Build history of the part. All positions in model axes, mm. Round coordinates to 2 decimals unless told otherwise and drop trailing zeros. Write each loop counter-clockwise with the first axis right and the second up, starting at its lowest first coordinate (ties: lowest second). Pieces come first, ordered by that corner, then holes.
from build123d import *

# Parameters (mm, degrees)
F0_W     = 25.4
F0_H     = 25.4
F0_W_2   = 22.098
F0_H_2   = 22.098
F1_DEPTH = 2133.6
F3_DEPTH = 25.401
F5_DEPTH = 25.401


with BuildPart() as f1:
    # F0 (on Right) → F1 (new body)
    with BuildSketch(Plane.YZ):
        with Locations((12.7, 12.7)):
            Rectangle(F0_W, F0_H)
        with Locations((12.7, 12.7)):
            Rectangle(F0_W_2, F0_H_2, mode=Mode.SUBTRACT)
    extrude(amount=F1_DEPTH)

    # F2 (on face) → F3 (cut, through all)
    with BuildSketch(Plane.XY.offset(25.4)):
        Polygon((2108.2, 25.4), (2133.6, 0), (2133.6, 25.4), align=None)
    extrude(amount=-F3_DEPTH, mode=Mode.SUBTRACT)

    # F4 (on face) → F5 (cut, through all)
    with BuildSketch(Plane.XY.offset(25.4)):
        Polygon((0, 25.4), (0, 0), (25.4, 25.4), align=None)
    extrude(amount=-F5_DEPTH, mode=Mode.SUBTRACT)


solid = f1.part
1) Slice it at A-A (y = 14). Write the cut outline in (x, z).
Results:
outline: (14, 0) - (2119.6, 0) - (2119.6, 1.65) - (14, 1.65) - close; (14, 23.75) - (2119.6, 23.75) - (2119.6, 25.4) - (14, 25.4) - close
2) Slice it at B-B (x = 1838.5). Write the cut outline in (y, z).
Results:
outline: (0, 0) - (25.4, 0) - (25.4, 25.4) - (0, 25.4) - close; hole (1.65, 1.65) - (23.75, 1.65) - (23.75, 23.75) - (1.65, 23.75) - close
3) Wall check: L1, parallel to Z at x = 489.5, y = 2; L2, parallel to X at y = 4.25, z = 24.25. Give the ranges that are in metal, low to high.
Results:
L1: z = 0 to 1.65, 23.75 to 25.4
L2: x = 4.25 to 2129.35
